Part print with two shaded views. Sizes in mm from the minimum x, y, z corner. A direction names the side the tool comes from. Round coordinates to 2 decimals unless told otherwise and drop trailing zeros. Order: outer loops, then holes, each group sorted by start corner. A loop starts at its lowest first (then second) coordinate and runs counter-clockwise, first axis right, second up. Notation, with made-up numbers: M -10.75,68 L 35.25,68 A14 cw 35.25,85 Z; hole C -36,1.5 d1. An arc over 180 degrees is marked long. Put each result on its own line as item: value.
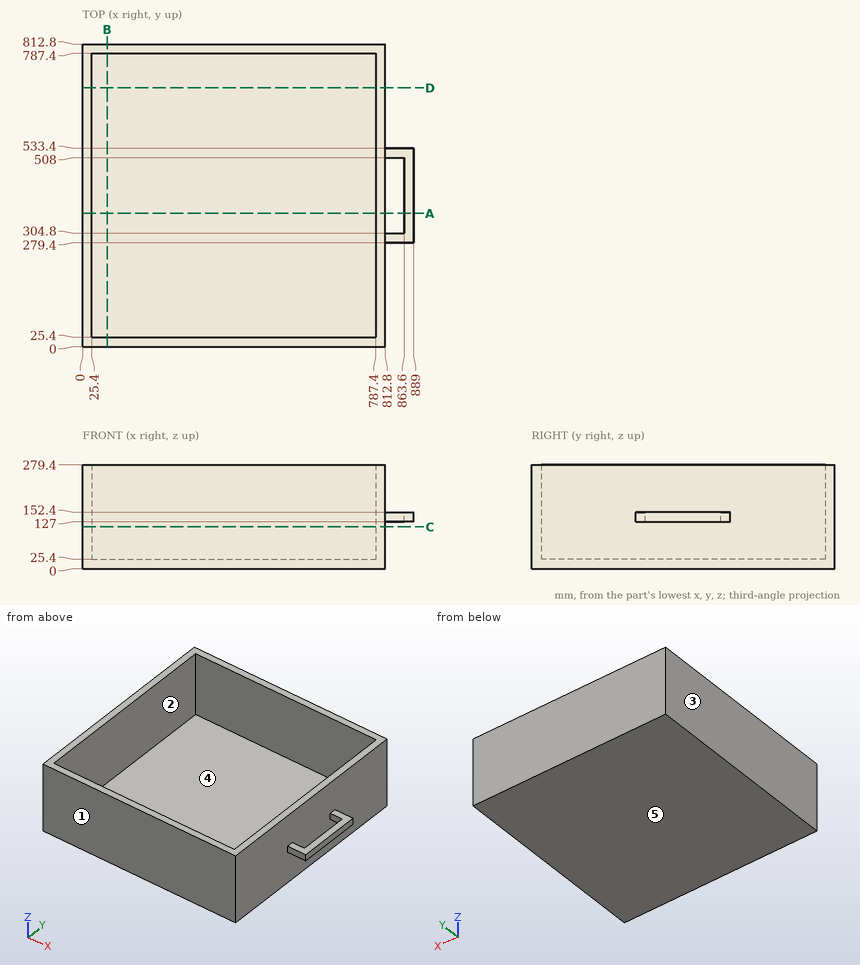
Item 1: Band-saw the part on B-B on x = 66. Give the cut face in (y, z), and give its area (3 significant figures).
Answers below:
outline: M 0,0 L 812.8,0 L 812.8,279.4 L 787.4,279.4 L 787.4,25.4 L 25.4,25.4 L 25.4,279.4 L 0,279.4 Z
area: 33,500 mm²
Item 2: Mould opens along X. For the marked faces 3, 4 and 5 say: pulls with the +X half, pulls with the -X half, needs draft (parallel to the pull), parting line crosses it, or undercut.
Answers below:
face 3: pulls with the -X half
face 4: undercut
face 5: needs draft
Item 3: Band-saw the part on A-A on y = 358. Give the cut face in (x, z).
Answers below:
outline: M 0,0 L 812.8,0 L 812.8,279.4 L 787.4,279.4 L 787.4,25.4 L 25.4,25.4 L 25.4,279.4 L 0,279.4 Z; M 863.6,127 L 889,127 L 889,152.4 L 863.6,152.4 Z
Item 4: Band-saw the part on C-C on z = 113. Give the cut face in (x, y).
Answers below:
outline: M 0,0 L 812.8,0 L 812.8,812.8 L 0,812.8 Z; hole M 25.4,25.4 L 787.4,25.4 L 787.4,787.4 L 25.4,787.4 Z
Item 5: Pin check, flat tips, straight feed: P1, Ø7.5, axis at x = 843.5, z = 136.5, coming from the +Y side; P2, Ø1.5, axis at y = 371.5, z = 36.5, coming from the +X side. Stop position of each tip, or through.
Answers below:
P1: y = 533.4
P2: x = 812.8
Item 6: Tool access for the marked faces 1 and 2: list every direction of +Z, -Z, +X, -X, +Y, -Y with a clear straight run to the whole face (end or side of a thin tool).
Answers below:
face 1: +Z, -Z, +X, -X, -Y
face 2: +Z
Item 7: Probe line 1 along Y through (x, z) = (334, 120); line 2 along Z through (x, y) = (439.5, 476). List the from-to ranges inside material, lowest first. Write a range as [from, to].
Answers below:
line 1: [0, 25.4], [787.4, 812.8]
line 2: [0, 25.4]
